Geometry: final body of the model. Coordinates: model frame, mm. A direction names the side the tool comes from. Give positions to 0.01 mm unless a question says otherwise; leave off trailing zeros. Write each loop counter-clockwise with the first axis right and the second up, starting at its lowest first coordinate (ties: lowest second). Pieces come first, ordered by that corner, then holes.
Q1. Reachability of faces 1 (the face through (24, -6, 2)), 2 (the face through (21, -14.9, 1)), 3 (the face through (7, 0, 2)) from +Z, -Z, +X, -X, +Y, -Y: full face, straight path, thin tool, end or side. Return the list, or none.
Q2. Cut plane C-C on x = 21. Return the cut outline in (y, z).
Q3. Cut plane B-B on y = -11.5. Return the cut outline in (x, z).
Q4. Draft query along Z for faces 4 (the face through (22, -21, 3.5)), 5 (the face through (16, -20, 0)), 6 (the face through (3.38, -2.96, 3.69)), 7 (the face through (21, -21.9, 1)). Return one class per face: pulls with the +Z half, pulls with the -Z half, needs draft (parallel to the pull), parting line crosses it, or undercut.
Q5. Cut plane D-D on y = -4. Return the cut outline in (x, z).
Q6. Cut plane A-A on z = 2.5. Return the cut outline in (x, y), plus the area to 3 significant figures.
Q7. Line query: L1, parallel to X at y = -5.5, z = 2.65; L2, parallel to X at y = -4.1, z = 2.5; L3, parallel to X at y = -26, z = 4.45. Output: solid intervals per line, ascending.
Q8. Pin query (flat end, axial travel): pin 1 (0.5 mm diameter, centred on y = -18.5, z = 1, fed in from +X); pin 2 (3.5 mm diameter, centred on x = 21, y = -19.4, fed in from -Z); pin 3 (1.2 mm diameter, centred on x = 24, z = 3, fed in from +Y). Return the tip coordinate at first contact, or that it passes through.
```python
from build123d import *

# Parameters (mm, degrees)
SKETCH_1_W                = 34
SKETCH_1_H                = 39.5
EXTRUDE_1_DEPTH           = 5
FILLET_1_R                = 12
SKETCH_2_R                = 3
CUT_EXTRUDE_2_DEPTH       = 5
SKETCH_3_R                = 4
CUT_EXTRUDE_3_DEPTH       = 5
SKETCH_4_R                = 5
CUT_EXTRUDE_4_DEPTH       = 4
CUT_EXTRUDE_5_DEPTH       = 10
EXTRUDE1_START            = -5
EXTRUDE1_DEPTH            = 5
SKETCH_8_R                = 1.5
CUT_EXTRUDE_6_DEPTH       = 4.5
SKETCH9_R                 = 0.5
EXTRUDE5_DEPTH            = 53.525447848
CUT_EXTRUDE_7_DEPTH       = 0.5
SKETCH_13_R               = 4
CUT_EXTRUDE_8_DEPTH       = 10
SKETCH2_W                 = 6
SKETCH2_H                 = 7
EXTRUDE2_DEPTH            = 2
HOLE_WIZARD_1_D           = 2.6
HOLE_WIZARD_1_CBORE_D     = 6
HOLE_WIZARD_1_CBORE_DEPTH = 1.5
SKETCH7_R                 = 1.5
EXTRUDE3_DEPTH            = 2
EXTRUDE4_DEPTH            = 53.570644581
SKETCH10_R                = 1.5
EXTRUDE6_DEPTH            = 10
CHAMFER_5_SIZE            = 0.1
SKETCH_22_R               = 1.5
EXTRUDE_1_2_DEPTH         = 5
CHAMFER_6_SIZE            = 0.5
SKETCH_5_R                = 1.25
CUT_EXTRUDE_1_DEPTH       = 6


with BuildPart() as part:
    # 草图1 → Extrude 1 (new body)
    with BuildSketch(Plane.XY):
        with Locations((17, -19.75)):
            Rectangle(SKETCH_1_W, SKETCH_1_H)
    extrude(amount=EXTRUDE_1_DEPTH)

    # 圆角1
    fillet_1_edges = [part.edges().sort_by_distance(p)[0] for p in [
        (0, -39.5, 2.5),
    ]]
    fillet(fillet_1_edges, radius=FILLET_1_R)

    # 草图2 → 拉伸2 (cut)
    with BuildSketch(Plane.XY.offset(5)):
        with Locations((26, -33.5)):
            Circle(SKETCH_2_R)
    extrude(amount=-CUT_EXTRUDE_2_DEPTH, mode=Mode.SUBTRACT)

    # 草图3 → 拉伸3 (cut)
    with BuildSketch(Plane(origin=(0, 0, 0), x_dir=(-1, 0, 0), z_dir=(0, 0, -1))):
        with Locations((-5.5, -11.5)):
            Circle(SKETCH_3_R)
    extrude(amount=-CUT_EXTRUDE_3_DEPTH, mode=Mode.SUBTRACT)

    # 草图4 → 拉伸4 (cut)
    with BuildSketch(Plane(origin=(0, 0, 0), x_dir=(-1, 0, 0), z_dir=(0, 0, -1))):
        with Locations((-5.5, -11.5)):
            Circle(SKETCH_4_R)
    extrude(amount=-CUT_EXTRUDE_4_DEPTH, mode=Mode.SUBTRACT)

    # 草图7 → 拉伸5 (cut)
    with BuildSketch(Plane(origin=(0, 0, 0), x_dir=(-1, 0, 0), z_dir=(0, 0, -1))):
        with BuildLine():
            Line((-26, -39.5), (-34, -39.5))
            Line((-34, -39.5), (-34, 0))
            Line((-34, 0), (-27.350847473, 0))
            Line((-27.350847473, 0), (-31.941608412, -32.664961394))
            ThreePointArc((-31.941608412, -32.664961394), (-30.528257481, -37.436354174), (-26, -39.5))
        make_face()
    extrude(amount=-CUT_EXTRUDE_5_DEPTH, mode=Mode.SUBTRACT)

    # Sketch1 → Extrude1 (add)
    with BuildSketch(Plane.XY.offset(5).offset(EXTRUDE1_START)):
        with BuildLine():
            Line((26.835038606, -39.441608412), (13.670077212, -41.291823076))
            ThreePointArc((13.670077212, -41.291823076), (4.127291652, -38.465121213), (0, -29.408606251))
            Line((0, -29.408606251), (0, -26.519790857))
            Line((0, -26.519790857), (29.441458618, -38.414912266))
            ThreePointArc((29.441458618, -38.414912266), (28.19900736, -39.082505408), (26.835038606, -39.441608412))
        make_face()
    extrude(amount=EXTRUDE1_DEPTH)

    # 草图8 → 拉伸6 (cut)
    with BuildSketch(Plane.XY.offset(5)):
        with Locations((2.5, -26.5)):
            Circle(SKETCH_8_R)
    extrude(amount=-CUT_EXTRUDE_6_DEPTH, mode=Mode.SUBTRACT)

    # Sketch9 → Extrude5 (cut, through all)
    with BuildSketch(Plane.XY.offset(0.5)):
        with Locations((1.5, -26.5)):
            Circle(SKETCH9_R)
    extrude(amount=-EXTRUDE5_DEPTH, mode=Mode.SUBTRACT)

    # 草图9 → 拉伸7 (cut)
    with BuildSketch(Plane.XY.offset(5)):
        with BuildLine():
            Line((0.25, -26.5), (0.25, -22.5))
            ThreePointArc((0.25, -22.5), (2.5, -20.25), (4.75, -22.5))
            Line((4.75, -22.5), (4.75, -26.5))
            ThreePointArc((4.75, -26.5), (2.5, -28.75), (0.25, -26.5))
        make_face()
    extrude(amount=-CUT_EXTRUDE_7_DEPTH, mode=Mode.SUBTRACT)

    # 草图13 → 拉伸8 (cut)
    with BuildSketch(Plane.XY.offset(5)):
        with Locations((16, -28.5)):
            Circle(SKETCH_13_R)
    extrude(amount=-CUT_EXTRUDE_8_DEPTH, mode=Mode.SUBTRACT)

    # Sketch2 → Extrude2 (cut)
    with BuildSketch(Plane(origin=(0, 0, 0), x_dir=(-1, 0, 0), z_dir=(0, 0, -1))):
        with Locations((-21, -18.4)):
            Rectangle(SKETCH2_W, SKETCH2_H)
    extrude(amount=-EXTRUDE2_DEPTH, mode=Mode.SUBTRACT)

    # 打孔尺寸(%根据)内六角圆柱头螺钉的类型1 (through all)
    with Locations(Plane(origin=(21, -19.4, 5), x_dir=(1, 0, 0), z_dir=(0, 0, 1))):
        with Locations((0, 0)):
            CounterBoreHole(HOLE_WIZARD_1_D / 2, HOLE_WIZARD_1_CBORE_D / 2, HOLE_WIZARD_1_CBORE_DEPTH)

    # Sketch7 → Extrude3 (cut)
    with BuildSketch(Plane(origin=(0, 0, 0), x_dir=(-1, 0, 0), z_dir=(0, 0, -1))):
        with Locations((-24, -16.4)):
            Circle(SKETCH7_R)
        with Locations((-18, -16.4)):
            Circle(SKETCH7_R)
        with Locations((-24, -20.4)):
            Circle(SKETCH7_R)
        with Locations((-18, -20.4)):
            Circle(SKETCH7_R)
    extrude(amount=-EXTRUDE3_DEPTH, mode=Mode.SUBTRACT)

    # Sketch8 → Extrude4 (cut, through all)
    with BuildSketch(Plane(origin=(0, 0, 0), x_dir=(-1, 0, 0), z_dir=(0, 0, -1))):
        with BuildLine():
            Line((-13.5, -6), (-13.5, 0))
            Line((-13.5, 0), (-18.5, 0))
            Line((-18.5, 0), (-18.5, -6))
            ThreePointArc((-18.5, -6), (-16, -8.5), (-13.5, -6))
        make_face()
    extrude(amount=-EXTRUDE4_DEPTH, mode=Mode.SUBTRACT)

    # Sketch10 → Extrude6 (cut)
    with BuildSketch(Plane.XY.offset(4.5)):
        with Locations((2.5, -26.5)):
            Circle(SKETCH10_R)
    extrude(amount=-EXTRUDE6_DEPTH, mode=Mode.SUBTRACT)

    # 倒角5
    chamfer_5_edges = [part.edges().sort_by_distance(p)[0] for p in [
        (10.5, -11.5, 0),
    ]]
    chamfer(chamfer_5_edges, length=CHAMFER_5_SIZE)

    # 草图22 → Extrude 1 2 (add)
    with BuildSketch(Plane.XY.offset(5)):
        with BuildLine():
            Line((4.75, -26.5), (4.75, -22.5))
            ThreePointArc((4.75, -22.5), (2.5, -20.25), (0.25, -22.5))
            Line((0.25, -22.5), (0.25, -26.5))
            ThreePointArc((0.25, -26.5), (2.5, -28.75), (4.75, -26.5))
        make_face()
        with Locations((2.5, -26.5)):
            Circle(SKETCH_22_R, mode=Mode.SUBTRACT)
    extrude(amount=-EXTRUDE_1_2_DEPTH)

    # 倒角6
    chamfer_6_edges = [part.edges().sort_by_distance(p)[0] for p in [
        (1, -26.5, 5),
    ]]
    chamfer(chamfer_6_edges, length=CHAMFER_6_SIZE)

    # 草图5 → 切除-拉伸1 (cut)
    with BuildSketch(Plane(origin=(0, 0, 0), x_dir=(1, 0, 0), z_dir=(0, 1, 0))):
        with Locations(Location((24, -2.5, 0), (0, 0, 270))):
            Circle(SKETCH_5_R)
        with Locations(Location((3, -2.5, 0), (0, 0, 270))):
            Circle(SKETCH_5_R)
    extrude(amount=-CUT_EXTRUDE_1_DEPTH, mode=Mode.SUBTRACT)


solid = part.part
```
Data:
1. face 1: +Y
1. face 2: -Z
1. face 3: +Z, -Z, +X, -X, +Y
2. outline: (-40.26, 0) - (-21.9, 0) - (-21.9, 2) - (-20.7, 2) - (-20.7, 3.5) - (-22.4, 3.5) - (-22.4, 5) - (-40.26, 5) - close; (-18.1, 2) - (-14.9, 2) - (-14.9, 0) - (0, 0) - (0, 5) - (-16.4, 5) - (-16.4, 3.5) - (-18.1, 3.5) - close
3. outline: (0, 0) - (0.4, 0) - (0.5, 0.1) - (0.5, 4) - (1.5, 4) - (1.5, 5) - (0, 5) - close; (9.5, 4) - (10.5, 4) - (10.5, 0.1) - (10.6, 0) - (28.97, 0) - (28.97, 5) - (9.5, 5) - close
4. face 4: pulls with the +Z half
4. face 5: pulls with the -Z half
4. face 6: undercut
4. face 7: needs draft
5. outline: (0, 0) - (13.5, 0) - (13.5, 5) - (0, 5) - close; (18.5, 0) - (27.91, 0) - (27.91, 5) - (18.5, 5) - close; hole circle Ø2.5 at (3, 2.5); hole circle Ø2.5 at (24, 2.5)
6. outline: (0, -29.41) arc R12 ccw to (13.67, -41.29) - (26.84, -39.44) arc R6 ccw to (31.94, -32.66) - (27.35, 0) - (25.25, 0) - (25.25, -6) - (22.75, -6) - (22.75, 0) - (18.5, 0) - (18.5, -6) arc R2.5 cw to (13.5, -6) - (13.5, 0) - (4.25, 0) - (4.25, -6) - (1.75, -6) - (1.75, 0) - (0, 0) - close; hole circle Ø10 at (5.5, -11.5); hole circle Ø3 at (2.5, -26.5); hole circle Ø8 at (16, -28.5); hole circle Ø2.6 at (21, -19.4); hole circle Ø6 at (26, -33.5)
6. area: 947 mm2
7. L1: x = 0 to 1.76, 4.24 to 13.5, 18.5 to 22.76, 25.24 to 28.12
7. L2: x = 0 to 1.75, 4.25 to 13.5, 18.5 to 22.75, 25.25 to 27.93
7. L3: x = 0 to 1.09, 3.91 to 12.88, 19.12 to 31
8. pin 1: stops at x = 29.99
8. pin 2: stops at z = 2
8. pin 3: stops at y = -6
